The drawing under review shows one solid part. Ordinate dimensions are in mm from its lowest x, y, z. Give positions to 0.01 mm unless a question says otherwise; leave off trailing zeros. Write each loop counter-clockwise with the first axis right and the second up, starting at its lowest first coordinate (ties: lowest second). Pieces come first, ordered by that corner, then holes. Notation, with made-up numbers: M 66,32 L 71,32 A16 ccw 71,38 Z; hole C -6,43 d10. An arc over 180 degrees is marked long. One line per item, written item: value. Start each with the question number.
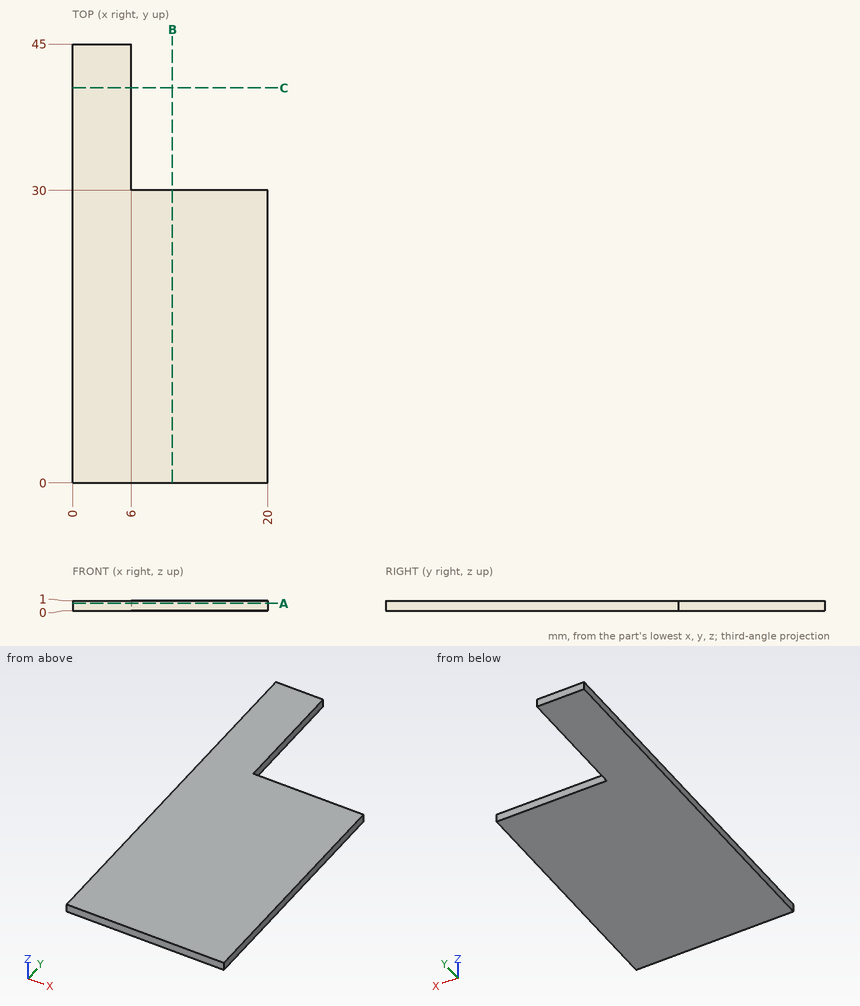
Q1. Wall thickness on line 1 (Y direction, x = 18.75, z = 0.4); line 2 (X direction, y = 41.5, z = 0.7): over which ranges is each line inside the solid? List them lowest first. Write a range as from..to.
Q2. Take a section at C-C, the plane y = 40.5. Give the boundary of the cut face in (x, z).
Q3. Take a section at A-A, the plane z = 0.75. Give the boundary of the cut face in (x, y).
Q4. For P1, Ø0.5, axis at x = 16.5, z = 0.5, coming from the +Y side, flat-tipped, find the tip position at first contact; note if it passes through.
Q5. Take a section at B-B, the plane x = 10.25. Give the boundary of the cut face in (y, z).
Results list:
1. line 1: y = 0..30
1. line 2: x = 0..6
2. outline: M 0,0 L 6,0 L 6,1 L 0,1 Z
3. outline: M 0,0 L 20,0 L 20,30 L 6,30 L 6,45 L 0,45 Z
4. P1: stops at y = 30
5. outline: M 0,0 L 30,0 L 30,1 L 0,1 Z
